Autodesk Inventor part; units mm, degrees
ref_plane "YZ Plane" through (0, 0, 0) normal (1, 0, 0) x (0, 1, 0)
ref_plane "XZ Plane" through (0, 0, 0) normal (0, 1, 0) x (-1, 0, 0)
ref_plane "XY Plane" through (0, 0, 0) normal (0, 0, 1) x (1, 0, 0)
sketch "Sketch1" plane through (0, 0, 0) normal (0, 0, 1) x (1, 0, 0)
  line L0 (-9.375, -11.75) -> (9.375, -11.75)
  line L1 (9.375, -11.75) -> (9.375, 11.75)
  line L2 (9.375, 11.75) -> (-9.375, 11.75)
  line L3 (-9.375, 11.75) -> (-9.375, -11.75)
  line L4 (-9.375, -11.75) -> (9.375, 11.75) construction
  line L5 (9.375, -11.75) -> (-9.375, 11.75) construction
  point P0 (0, 0)
  dimension "d0" = 18.75
  dimension "d1" = 23.5
extrude "Extrusion1" add sketch "Sketch1" along normal blind 28.5
sketch "Sketch2" plane through (-9.375, 11.75, 0) normal (0, 1, 0) x (1, 0, 0)
  line L0 (0, -28.5) -> (18.75, -28.5)
  line L1 (0, -28.5) -> (4.75, -28.5)
  line L2 (18.75, 0) -> (18.75, -9.5)
  line L3 (18.75, 0) -> (18.75, -28.5)
  line L4 (18.75, -9.5) -> (4.75, -28.5)
  line L5 (18.75, -28.5) -> (4.75, -28.5)
  line L6 (18.75, -28.5) -> (18.75, -9.5)
  point P0 (9.375, 0)
  dimension "d4" = 4.75
  dimension "d5" = 9.5
extrude "Extrusion2" cut sketch "Sketch2" against normal blind 28.5
sketch "Sketch7" plane through (-9.375, 11.75, 0) normal (0, 1, 0) x (1, 0, 0)
  line L0 (18.75, 0) -> (18.75, -9.5)
  line L1 (18.75, -9.5) -> (18.75, 0)
  line L2 (18.75, 0) -> (14.25, 0)
  line L3 (0, 0) -> (18.75, 0)
  line L4 (14.25, 0) -> (14.25, -15.6071)
  line L5 (18.75, -9.5) -> (4.75, -28.5)
  line L6 (18.75, -9.5) -> (14.25, -15.6071)
  point P0 (9.375, 0)
  dimension "d27" = 4.5
extrude "Extrusion7" cut sketch "Sketch7" against normal blind 4.5
sketch "Sketch8" plane through (-9.375, -11.75, 0) normal (0, -1, 0) x (1, 0, 0)
  line L0 (18.75, 0) -> (18.75, 9.5)
  line L1 (18.75, 0) -> (14.25, 0)
  line L2 (0, 0) -> (18.75, 0)
  line L3 (18.75, 9.5) -> (14.25, 15.6071)
  line L4 (14.25, 0) -> (14.25, 15.6071)
  line L5 (14.25, 15.6071) -> (18.75, 9.5)
  line L6 (18.75, 0) -> (18.75, 9.5)
  point P0 (9.375, 0)
  dimension "d30" = 4.5
extrude "Extrusion8" cut sketch "Sketch8" against normal blind 4.5
sketch "Sketch9" plane through (-9.375, -11.75, 0) normal (-1, 0, 0) x (0, 0, 1)
  line L0 (15.6071, 19) -> (0, 19)
  line L1 (28.5, 4.5) -> (0, 4.5)
  line L2 (0, 4.5) -> (0, 19)
  line L3 (0, 19) -> (28.5, 19)
  line L4 (28.5, 19) -> (28.5, 4.5)
  line L5 (28.5, 23.5) -> (28.5, 0)
  line L6 (0, 0) -> (28.5, 0)
  point P0 (0, 11.75)
  dimension "d35" = 0
  dimension "d36" = 4.5
extrude "Extrusion9" cut sketch "Sketch9" against normal blind 9.5
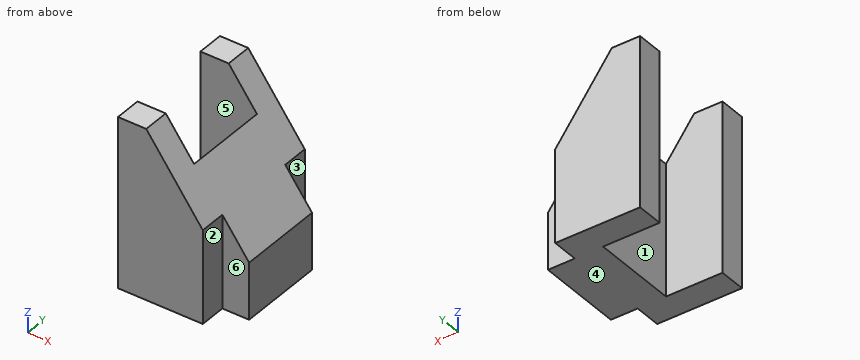
Work out the finished part from the listing and answer in its coordinate system (mm). Face numbers are marked on the shaded views. A direction names the side the tool comes from. Round coordinates to 2 decimals unless told otherwise and drop trailing zeros. Loops run counter-clockwise (first coordinate to the right, second up) from the corner with the lowest first, then second, coordinate; pieces in that order, holes last.
(1) The part is cut by section B-B, the plane z = 23. Give the vertices of the cut face in (x, y) (3 decimals), and give its area (3 significant figures).
Computed values:
outline: (-9.375, -11.75) - (-0.572, -11.75) - (-0.572, -7.25) - (-9.375, -7.25) - close; (-9.375, 7.25) - (-0.572, 7.25) - (-0.572, 11.75) - (-9.375, 11.75) - close
area: 79.2 mm2
(2) The part is cut by section D-D, the plane y = -4.5. Give the vertices of the cut face in (x, z) (3 decimals).
Computed values:
outline: (0.125, 0) - (9.375, 0) - (9.375, 9.5) - (0.125, 22.054) - close
(3) The mould has two halves that part along Y. Classify the marked faces 4, 5 and 6: pulls with the +Y half, pulls with the -Y half, needs draft (parallel to the pull), parting line crosses it, or undercut.
Computed values:
face 4: needs draft
face 5: undercut
face 6: pulls with the -Y half
(4) For the marked faces 1, 2 and 3, determine the directions among +Z, -Z, +X, -X, +Y, -Y from which every point of the face is accessible in a straight line to the end or side of a thin tool.
Computed values:
face 1: +Z, -Z, -X
face 2: +Z, -Z, +X, -Y
face 3: +Z, -Z, +X, +Y
(5) Each of these flat-tipped pins is pushed along its axis until it touches: P1, Ø3, axis at y = 4, z = 3.5, coming from the -X side (3 decimals); P2, Ø5, axis at y = -10, z = 8, coming from the +X side (3 decimals); P3, Ø1.4, axis at x = 8, z = 9, coming from the -Y side. Where does it stop, or does it pass through?
Computed values:
P1: stops at x = 0.125
P2: stops at x = 4.875
P3: stops at y = -7.25
(6) The part is cut by section A-A, the plane x = -7.5. Give the vertices of the cut face in (y, z).
Computed values:
outline: (-11.75, 0) - (-7.25, 0) - (-7.25, 28.5) - (-11.75, 28.5) - close; (7.25, 0) - (11.75, 0) - (11.75, 28.5) - (7.25, 28.5) - close
(7) Find the intervals of material crossed by L1, parallel to Y at x = -3.5, z = 20.75; L2, parallel to X at y = 10, z = 12.75 (3 decimals); L3, parallel to X at y = 4.25, z = 8.5 (3 decimals), in increasing order.
Computed values:
L1: y = -11.75 to -7.25, 7.25 to 11.75
L2: x = -9.375 to 4.875
L3: x = 0.125 to 9.375
(8) The part is cut by section C-C, the plane z = 5.25. Give the vertices of the cut face in (x, y) (3 decimals), and give its area (3 significant figures).
Computed values:
outline: (-9.375, -11.75) - (4.875, -11.75) - (4.875, -7.25) - (9.375, -7.25) - (9.375, 7.25) - (4.875, 7.25) - (4.875, 11.75) - (-9.375, 11.75) - (-9.375, 7.25) - (0.125, 7.25) - (0.125, -7.25) - (-9.375, -7.25) - close
area: 262 mm2
